Read the model definition and answer for the solid it produces. Units are mm, in the model's axes. Face numbers are marked on the shaded views. A direction names the side the tool comes from. Give positions to 0.01 mm unless a question says otherwise; leave off trailing zeros. Write each loop counter-clockwise with the first axis right and the second up, starting at its lowest first coordinate (ties: lowest second). Pieces come first, ordered by that corner, then holes.
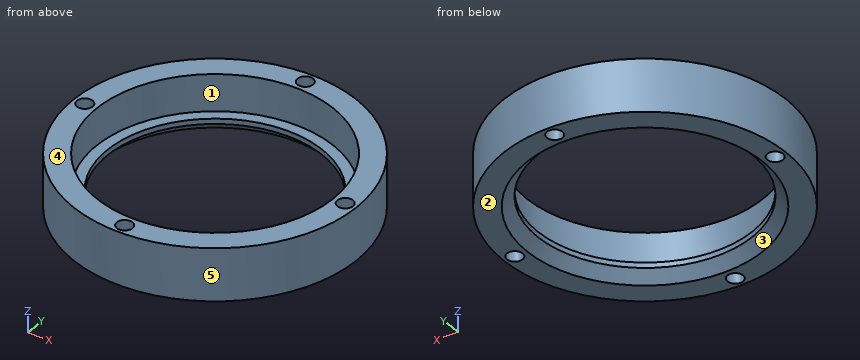
```python
from build123d import *

# Parameters (mm, degrees)
F0_R     = 27
F1_DEPTH = 10
F2_R     = 22.6
F3_DEPTH = 7
F4_R     = 20.5
F5_DEPTH = 3.001
F6_R     = 1.5
F7_DEPTH = 10.001
F8_SIZE  = 2


with BuildPart() as f1:
    # F0 (on Top) → F1 (new body)
    with BuildSketch(Plane.XY):
        Circle(F0_R)
    extrude(amount=F1_DEPTH)

    # F2 (on face) → F3 (cut)
    with BuildSketch(Plane.XY.offset(10)):
        Circle(F2_R)
    extrude(amount=-F3_DEPTH, mode=Mode.SUBTRACT)

    # F4 (on face) → F5 (cut, through all)
    with BuildSketch(Plane.XY.offset(3)):
        Circle(F4_R)
    extrude(amount=-F5_DEPTH, mode=Mode.SUBTRACT)

    # F6 (on face) → F7 (cut, through all)
    with BuildSketch(Plane.XY.offset(10)):
        with Locations((-24.875, 0)):
            Circle(F6_R)
        with Locations((24.875, 0)):
            Circle(F6_R)
        with Locations((0, 24.875)):
            Circle(F6_R)
        with Locations((0, -24.875)):
            Circle(F6_R)
    extrude(amount=-F7_DEPTH, mode=Mode.SUBTRACT)

    # F8
    f8_edges = [f1.edges().sort_by_distance(p)[0] for p in [
        (-20.5, 0, 0),
    ]]
    chamfer(f8_edges, length=F8_SIZE)


solid = f1.part
```
Item 1: Find the intervals of material crossed by line 1 along Y through (x, z) = (0, 2.45) (3 decimals); line 2 along Y through (x, z) = (1, 8.25); line 3 along Y through (x, z) = (17, 6.5), in increasing order.
Result set:
line 1: y = -27 to -26.375, -23.375 to -20.5, 20.5 to 23.375, 26.375 to 27
line 2: y = -26.98 to -25.99, -23.76 to -22.58, 22.58 to 23.76, 25.99 to 26.98
line 3: y = -20.98 to -14.89, 14.89 to 20.98
Item 2: Determine the mould class of the marked faces 3, 4 and 5 for opening direction X: pulls with the +X half, pulls with the -X half, needs draft (parallel to the pull), parting line crosses it, or undercut.
Result set:
face 3: undercut
face 4: needs draft
face 5: parting line crosses it
Item 3: Section A-A (x = 0) is taken. Write down the section's boundary in (y, z) (3 decimals).
Result set:
outline: (-27, 0) - (-26.375, 0) - (-26.375, 10) - (-27, 10) - close; (-23.375, 0) - (-22.5, 0) - (-20.5, 2) - (-20.5, 3) - (-22.6, 3) - (-22.6, 10) - (-23.375, 10) - close; (20.5, 2) - (22.5, 0) - (23.375, 0) - (23.375, 10) - (22.6, 10) - (22.6, 3) - (20.5, 3) - close; (26.375, 0) - (27, 0) - (27, 10) - (26.375, 10) - close
Item 4: Each of these flat-tipped pins is pushed along its axis until it touches: pin 1 Ø1.5 at (y, z) = (4, 7) entering from -X; pin 2 Ø1.5 at (y, z) = (4, 4) entering from +X; pin 3 Ø1 at (x, z) = (11.5, 7) entering from -Y. Where does it stop, or does it pass through?
Result set:
pin 1: stops at x = -26.8
pin 2: stops at x = 26.8
pin 3: stops at y = -24.66
Item 5: Which of the six approach directions +Z, -Z, +X, -X, +Y, -Y give full straight-line access (tool end or side, diameter ignored) to the marked faces 1 and 2?
Result set:
face 1: +Z
face 2: -Z, +X, -X, +Y, -Y
Item 6: Section C-C (z = 4.5) is taken. Write down the section's boundary in (x, y) (3 decimals), and give its area (3 significant figures).
Result set:
outline: circle Ø54 at (0, 0); hole circle Ø3 at (-24.875, 0); hole circle Ø45.2 at (0, 0); hole circle Ø3 at (0, -24.875); hole circle Ø3 at (0, 24.875); hole circle Ø3 at (24.875, 0)
area: 657 mm2
